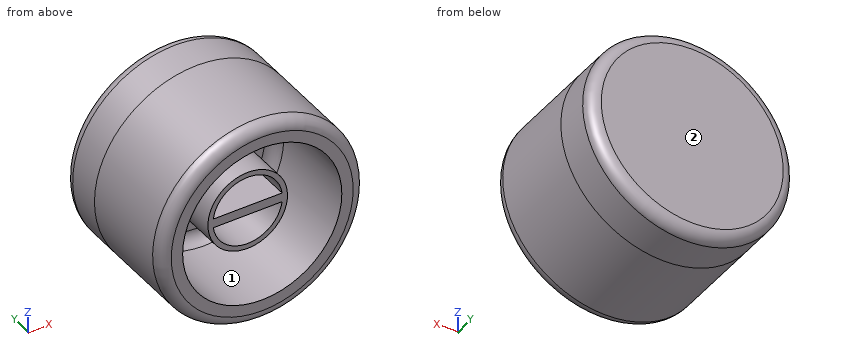
from build123d import *

# Parameters (mm, degrees)
SKETCH1_R           = 3.5
BOSS_EXTRUDE1_DEPTH = 7
SKETCH2_R           = 9
BOSS_EXTRUDE2_DEPTH = 4
BOSS_EXTRUDE3_START = 9
SKETCH3_R           = 9
SKETCH3_R_2         = 7
BOSS_EXTRUDE3_DEPTH = 9
FILLET1_R           = 1


with BuildPart() as part:
    # Sketch1 → Boss-Extrude1 (new body)
    with BuildSketch(Plane(origin=(0, 0, 0), x_dir=(1, 0, 0), z_dir=(0, 1, 0))):
        with Locations(Location((0, 0, 0), (0, 0, 270))):
            Circle(SKETCH1_R)
        with BuildLine():
            Line((3.023656727, 0.4), (-3.023656727, 0.4))
            ThreePointArc((-3.023656727, 0.4), (0, 3.05), (3.023656727, 0.4))
        make_face(mode=Mode.SUBTRACT)
        with BuildLine():
            Line((-3.023656727, -0.4), (3.023656727, -0.4))
            ThreePointArc((3.023656727, -0.4), (0, -3.05), (-3.023656727, -0.4))
        make_face(mode=Mode.SUBTRACT)
    extrude(amount=BOSS_EXTRUDE1_DEPTH)

    # Sketch2 → Boss-Extrude2 (add)
    with BuildSketch(Plane(origin=(0, 7, 0), x_dir=(1, 0, 0), z_dir=(0, 1, 0))):
        with Locations(Location((0, 0, 0), (0, 0, 270))):
            Circle(SKETCH2_R)
    extrude(amount=BOSS_EXTRUDE2_DEPTH)

    # Sketch3 → Boss-Extrude3 (add)
    with BuildSketch(Plane.XZ.offset(-7).offset(BOSS_EXTRUDE3_START)):
        with Locations(Location((0, 0, 0), (0, 0, 270))):
            Circle(SKETCH3_R)
        with Locations(Location((0, 0, 0), (0, 0, 270))):
            Circle(SKETCH3_R_2, mode=Mode.SUBTRACT)
    extrude(amount=-BOSS_EXTRUDE3_DEPTH)

    # Fillet1
    fillet1_edges = [part.edges().sort_by_distance(p)[0] for p in [
        (0, 11, -9),
        (0, 7, -3.5),
        (0, -2, 9),
        (0, 7, 7),
    ]]
    fillet(fillet1_edges, radius=FILLET1_R)


solid = part.part
Can you work these out from the model? Positions are in its coordinate system, mm. Face numbers are marked on the shaded views. Give positions to 0.01 mm unless a question says otherwise; leave off trailing zeros. Order: outer loops, then holes, each group sorted by start corner. A loop starts at its lowest first (then second) coordinate and runs counter-clockwise, first axis right, second up. Notation, with made-up numbers: M 81.25,-1 L 134.25,-1 A14 ccw 134.25,19 Z; hole C -8,-17.75 d11. An arc over 180 degrees is marked long. Use one line per item in the form item = value. Start each with the question number.
Item 1: If we section it at A-A (y = 1.5): Write out the boundary of the cut face in (x, z), then the cut area to 3 significant figures.
Item 2: If I drill on line 1 along X through (y, z) = (0.75, 0); line 2 along X through (y, z) = (-0.5, 0); line 3 along X through (y, z) = (6.75, -2.25), over which ranges is the centre line in solid material (lowest first)?
Item 3: Will these pins go through, and if not, where does the flat tip stop? pin 1 Ø6 at (x, y) = (5.5, 1.5) entering from -Z; pin 2 Ø3.5 at (x, z) = (1.5, 0) entering from -Y; pin 3 Ø2 at (x, z) = (0, -1.5) entering from -Y.
Item 4: If we section it at B-B (z = 0): Write out the boundary of the cut face in (x, y), then the cut area to 3 significant figures.
Item 5: If we section it at D-D (y = 6.5): Write out the boundary of the cut face in (x, z), then the cut area to 3 significant figures.
Item 6: We'd pull the mould along Z, two halves only. Please class the marked faces 1 and 2: +Z half, -Z half, draft (parallel to the pull), parting line (faces both ways), or undercut.
Item 7: If we section it at C-C (x = 0): Write out the boundary of the cut face in (y, z).
Outcome:
q1.outline = C 0,0 d18; C 0,0 d7; hole C 0,0 d14; hole M -3.02,-0.4 A3.05 ccw 3.02,-0.4 Z; hole M -3.02,0.4 L 3.02,0.4 A3.05 ccw Z
q1.area = 115 mm2
q2.line_1 = -9 to -7, -3.5 to 3.5, 7 to 9
q2.line_2 = -9 to -7, 7 to 9
q2.line_3 = -8.71 to -6.27, -3.11 to -2.06, 2.06 to 3.11, 6.27 to 8.71
q3.pin_1 = -8.65
q3.pin_2 = 0
q3.pin_3 = 7
q4.outline = M -9,-1 A1 ccw -8,-2 L -7,-2 L -7,6 A1 cw -6,7 L -4.5,7 A1 cw -3.5,6 L -3.5,0 L 3.5,0 L 3.5,6 A1 cw 4.5,7 L 6,7 A1 cw 7,6 L 7,-2 L 8,-2 A1 ccw 9,-1 L 9,10 A1 ccw 8,11 L -8,11 A1 ccw -9,10 Z
q4.area = 157 mm2
q5.outline = C 0,0 d18; C 0,0 d7.27; hole C 0,0 d13.73; hole M -3.02,-0.4 A3.05 ccw 3.02,-0.4 Z; hole M -3.02,0.4 L 3.02,0.4 A3.05 ccw Z
q5.area = 123 mm2
q6.face_1 = undercut
q6.face_2 = draft
q7.outline = M -2,-8 A1 ccw -1,-9 L 10,-9 A1 ccw 11,-8 L 11,8 A1 ccw 10,9 L -1,9 A1 ccw -2,8 L -2,7 L 6,7 A1 cw 7,6 L 7,4.5 A1 cw 6,3.5 L 0,3.5 L 0,3.05 L 7,3.05 L 7,0.4 L 0,0.4 L 0,-0.4 L 7,-0.4 L 7,-3.05 L 0,-3.05 L 0,-3.5 L 6,-3.5 A1 cw 7,-4.5 L 7,-6 A1 cw 6,-7 L -2,-7 Z
